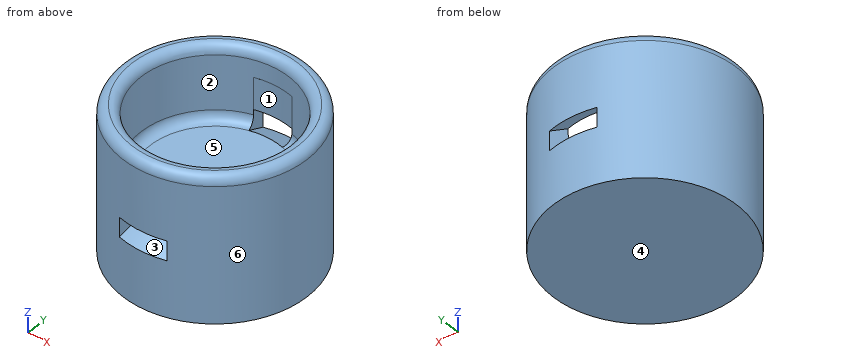
```python
from build123d import *

# Parameters (mm, degrees)
F1_R          = 16.129
F2_DEPTH      = 25.4
F3_R          = 12.954
F4_DEPTH      = 12.7
F5_R          = 1.58749
F7_ANGLE_BACK = 15
F7_ANGLE      = 30
F8_T4_ANGLE   = 47.2856392703
F8_S5_R       = 12.954
F8_T6_DEPTH   = 7
F8_T10_ANGLE  = 47.2856392703
F8_S11_R      = 12.954
F8_T12_DEPTH  = 7


# Not quite as in the source:
# - a fillet or chamfer that OpenCascade refuses, or shapes differently, is made with other operations: its cross-section is extruded or revolved along the edge and cut away or added
# - a fillet or chamfer is up to 0.001 mm smaller than in the source, because OpenCascade refuses the exact size
# - ends of sketch curves that miss each other by under 0.0002 mm in the source are joined


with BuildPart() as f2:
    # F1 (on Top) → F2 (new body)
    with BuildSketch(Plane.XY):
        Circle(F1_R)
    extrude(amount=F2_DEPTH)

    # F3 (on face) → F4 (cut)
    with BuildSketch(Plane.XY.offset(25.4)):
        Circle(F3_R)
    extrude(amount=-F4_DEPTH, mode=Mode.SUBTRACT)

    # F5 (radius 1.5875 in the source; OpenCascade refuses exactly that, so slightly less here)
    f5_edges = [f2.edges().sort_by_distance(p)[0] for p in [
        (-16.129, 0, 25.4),
        (-12.954, 0, 25.4),
        (-12.954, 0, 12.7),
    ]]
    fillet(f5_edges, radius=F5_R)

    # F6 (on Right) → F7 (revolve, cut)
    with BuildSketch(Plane.YZ, mode=Mode.PRIVATE) as f7_sk:
        with BuildLine():
            ThreePointArc((12.2294899884, 15.6199430682), (12.8889010018, 13.8375539592), (11.3665, 12.7))
            Line((11.3665, 12.7), (16.129, 9.8708188202))
            Line((16.129, 9.8708188202), (16.129, 13.3034244871))
            Line((16.129, 13.3034244871), (12.9914900466, 15.1672741693))
            Line((12.9914900466, 15.1672741693), (12.2294899884, 15.6199430682))
        make_face()
        with BuildLine():
            Line((-16.129, 9.8708188202), (-11.3665, 12.7))
            ThreePointArc((-11.3665, 12.7), (-12.8889010018, 13.8375539592), (-12.2294899884, 15.6199430682))
            Line((-12.2294899884, 15.6199430682), (-12.9914900466, 15.1672741693))
            Line((-12.9914900466, 15.1672741693), (-16.129, 13.3034244871))
            Line((-16.129, 13.3034244871), (-16.129, 9.8708188202))
        make_face()
        Polygon((12.2294900466, 21.5172741693), (12.2294900466, 15.6199431581), (12.9914900466, 15.1672741693), (12.9914900466, 21.5172741693), align=None)
        Polygon((-12.9914900466, 15.1672741693), (-12.2294900466, 15.6199431581), (-12.2294900466, 21.5172741693), (-12.9914900466, 21.5172741693), align=None)
    revolve(f7_sk.sketch.rotate(Axis((0, 0, 7.0286970586), (0, 0, -1)), -F7_ANGLE_BACK), axis=Axis((0, 0, 7.0286970586), (0, 0, -1)), revolution_arc=F7_ANGLE, mode=Mode.SUBTRACT)

    # F8: chamfer of 0.762 on 2 edges, made by hand


with BuildPart() as f8_tool2:
    # F8_s3 → F8_t4 (revolve)
    with BuildSketch(Plane(origin=(0, 0, 0), x_dir=(0, 0, 1), z_dir=(0.9160632754, 0.4010337585, 0))):
        Polygon((21.5172741693, 12.2294900466), (20.7552741693, 12.9914900466), (21.5172741693, 12.9914900466), align=None)
    revolve(axis=Axis((0, 0, 21.5172741693), (0, 0, -1)), revolution_arc=F8_T4_ANGLE)

    # F8_s5 → F8_t6 (cut, symmetric)
    with BuildSketch(Plane.XY.offset(21.1)):
        Circle(F8_S5_R)
    extrude(amount=F8_T6_DEPTH, both=True, mode=Mode.SUBTRACT)


with BuildPart() as f2_1:
    add(f2.part)

    # F8_t1: union F8_tool2
    add(f8_tool2.part)


with BuildPart() as f8_tool8:
    # F8_s9 → F8_t10 (revolve)
    with BuildSketch(Plane(origin=(0, 0, 0), x_dir=(0, 0, 1), z_dir=(-0.9160632754, -0.4010337585, 0))):
        Polygon((21.5172741693, 12.2294900466), (20.7552741693, 12.9914900466), (21.5172741693, 12.9914900466), align=None)
    revolve(axis=Axis((0, 0, 21.5172741693), (0, 0, -1)), revolution_arc=F8_T10_ANGLE)

    # F8_s11 → F8_t12 (cut, symmetric)
    with BuildSketch(Plane.XY.offset(21.1)):
        Circle(F8_S11_R)
    extrude(amount=F8_T12_DEPTH, both=True, mode=Mode.SUBTRACT)


with BuildPart() as f2_2:
    add(f2_1.part)

    # F8_t7: union F8_tool8
    add(f8_tool8.part)


solid = f2_2.part
```
Build history of the part. All positions in model axes, mm. Face numbers are marked on the shaded views. A direction names the side the tool comes from. Give positions to 0.01 mm unless a question says otherwise; leave off trailing zeros. Loops run counter-clockwise (first coordinate to the right, second up) from the corner with the lowest first, then second, coordinate; pieces in that order, holes last. Notation, with made-up numbers: (-2.5, 41.5) -> (25.5, 41.5) arc R35 ccw to (25.5, 74.5) -> close; hole circle Ø10 at (-29.5, 63.5). An arc over 180 degrees is marked (long way). One line per question, with ' | ' between items. Start each with the question number.
1) Cut at D-D (z = 5.5). Give the cut face in (x, y), plus the area to 3 significant figures.
2) Pin check, flat tips, straight feed: pin 1 (1.5 mm diameter, centred on y = 6, z = 11, fed in from +X); pin 2 (10 mm diameter, centred on x = -6.5, z = 21.5, fed in from +Y); pin 3 (2 mm diameter, centred on x = -12, z = 19, fed in from +Y). Stop position of each tip, or through.
3) Cut at A-A (x = 0). Count the separate pieces of the cut face and the enclosed holes in it, plus the area to 3 significant figures.
4) Two-plate mould, pull along Y, no slides. Class the marked faces 4, 5 and 6: released by +Y, released by -Y, zero draft, split by the parting line, or undercut.
5) Cut at C-C (z = 21.5). Give the cut face in (x, y).
6) Probe L1, parallel to Y at x = 0, z = 21; L2, parallel to X at y = -11, z = 15.75; L3, parallel to Z at x = -3, y = -3. List the from-to ranges inside material, lowest first.
7) 3-axis set-ups, long thin cutter, end or side, ignore diameter. For the marked faces 1, 2 and 3: which of +Z, -Z, +X, -X, +Y, -Y reach the whole face in a straight line?
Return value:
1) outline: circle Ø32.26 at (0, 0) | area: 817 mm^2
2) pin 1: x = 15.25 | pin 2: y = 16.06 | pin 3: y = 11.8
3) separate pieces: 3 | enclosed holes: 0 | area: 464 mm^2
4) face 4: zero draft | face 5: undercut | face 6: split by the parting line
5) outline: circle Ø32.26 at (0, 0); hole circle Ø25.91 at (0, 0)
6) L1: -16.13 to -12.95, 12.95 to 16.13 | L2: -11.8 to -6.84, 6.84 to 11.8 | L3: 0 to 12.7
7) face 1: none | face 2: +Z | face 3: -Y
